Verification items for the finished model (mm, model axes). Face numbers are marked on the shaded views. A direction names the side the tool comes from. Give positions to 0.01 mm unless a question says otherwise; leave off trailing zeros. Write each loop counter-clockwise with the first axis right and the second up, starting at its lowest first coordinate (ties: lowest second). Pieces come first, ordered by that corner, then holes. Notation, with made-up numbers: (48.25, 7.25) - (91.25, 7.25) arc R13 ccw to (91.25, 16.25) - close; hole circle Ø7 at (-9, -1). An arc over 180 degrees is marked (long way). Put each result on its own line as item: value.
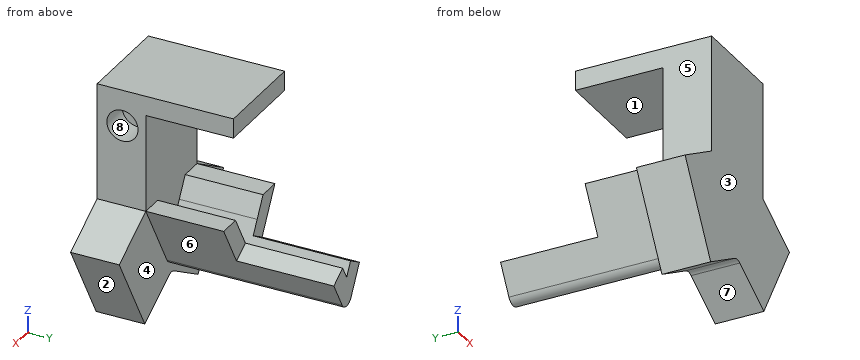
from build123d import *

# Parameters (mm, degrees)
BOSS_EXTRUDE1_DEPTH      = 2
BOSS_EXTRUDE1_DEPTH_BACK = 3
BOSS_EXTRUDE2_DEPTH      = 18
BOSS_EXTRUDE3_DEPTH      = 2
BOSS_EXTRUDE3_DEPTH_BACK = 3
SKETCH8_W                = 10
SKETCH8_H                = 12
SKETCH9_W                = 10
SKETCH9_H                = 2.002012711
BOSS_EXTRUDE4_DEPTH      = 18
CUT_EXTRUDE1_DEPTH       = 10
SKETCH12_W               = 10
SKETCH12_H               = 9
CUT_EXTRUDE3_DEPTH       = 3
FILLET3_R                = 1
FILLET4_R                = 1
SKETCH14_R               = 1.6
CUT_EXTRUDE4_DEPTH       = 3


with BuildPart() as part:
    # Sketch3 → Boss-Extrude1 (new, two sides: drawn at the far end of the back side and taken through both)
    with BuildSketch(Plane(origin=(0, 0, 0), x_dir=(1, 0, 0), z_dir=(0, 1, 0)).offset(-BOSS_EXTRUDE1_DEPTH_BACK)):
        Polygon((-16.281996431, 0), (-6.281996431, 0), (-1.085844009, 3), (-6.085844009, 11.660254038), (-11.281996431, 8.660254038), (-16.478148854, 11.660254038), (-21.478148854, 3), align=None)
    extrude(amount=BOSS_EXTRUDE1_DEPTH + BOSS_EXTRUDE1_DEPTH_BACK)

    # Sketch7 → Boss-Extrude2 (add)
    with BuildSketch(Plane(origin=(0, 2, 0), x_dir=(1, 0, 0), z_dir=(0, 1, 0))):
        Polygon((-6.281996431, 0), (-11.281996431, 8.660254038), (-16.281996431, 0), (-13.972595355, 0), (-12.817894816, 2), (-11.281996431, 4.660254038), (-9.746098047, 2), (-8.591397508, 0), align=None)
    extrude(amount=BOSS_EXTRUDE2_DEPTH)

    # Sketch8 → Boss-Extrude3 (add, two sides: drawn at the far end of the back side and taken through both)
    with BuildSketch(Plane(origin=(0, 0, 0), x_dir=(1, 0, 0), z_dir=(0, 1, 0)).offset(-BOSS_EXTRUDE3_DEPTH_BACK)):
        with Locations((-11.281996431, -6)):
            Rectangle(SKETCH8_W, SKETCH8_H)
    extrude(amount=BOSS_EXTRUDE3_DEPTH + BOSS_EXTRUDE3_DEPTH_BACK)

    # Sketch9 → Boss-Extrude4 (add)
    with BuildSketch(Plane(origin=(0, 2, 0), x_dir=(1, 0, 0), z_dir=(0, 1, 0))):
        with Locations((-11.281996431, -10.998993645)):
            Rectangle(SKETCH9_W, SKETCH9_H)
    extrude(amount=BOSS_EXTRUDE4_DEPTH)

    # Sketch10 → Cut-Extrude1 (cut)
    with BuildSketch(Plane(origin=(0, 20, 0), x_dir=(1, 0, 0), z_dir=(0, 1, 0))):
        Polygon((-13.781996431, 4.330127019), (-16.281996431, 0), (-13.972595355, 0), (-12.049945624, 3.330127019), align=None)
        Polygon((-6.281996431, 0), (-8.781996431, 4.330127019), (-10.514047239, 3.330127019), (-8.591397508, 0), align=None)
    extrude(amount=-CUT_EXTRUDE1_DEPTH, mode=Mode.SUBTRACT)

    # Sketch12 → Cut-Extrude3 (cut)
    with BuildSketch(Plane.XY.offset(12)):
        with Locations((-11.281996431, 15.5)):
            Rectangle(SKETCH12_W, SKETCH12_H)
    extrude(amount=-CUT_EXTRUDE3_DEPTH, mode=Mode.SUBTRACT)

    # Fillet3
    # the kernel refuses this fillet: 1 mm, written as the material it takes off along each edge
    with BuildSketch(Plane(origin=(-11.281996431, 2, -8.660254038), x_dir=(-0.5000000000000031, 0, 0.8660254037844368), z_dir=(0, 1, 0))) as fillet3_piece_1:
        with BuildLine():
            CenterArc((FILLET3_R * 1.73205080757, FILLET3_R), FILLET3_R, 150, 120)
            Line((FILLET3_R * 0.866025403784, FILLET3_R * 1.5), (0, 0))
            Line((0, 0), (FILLET3_R * 1.73205080757, 0))
        make_face()
    extrude(amount=22.330127019, mode=Mode.SUBTRACT)

    # Fillet4
    fillet4_edges = [part.edges().sort_by_distance(p)[0] for p in [
        (-11.281996431, -0.5, -8.660254038),
    ]]
    fillet(fillet4_edges, radius=FILLET4_R)

    # Sketch14 → Cut-Extrude4 (cut)
    with BuildSketch(Plane(origin=(-6.281996431, 0, 0), x_dir=(0, 0, -1), z_dir=(1, 0, 0))):
        with Locations((-8.29856454, -0.4)):
            Circle(SKETCH14_R)
    extrude(amount=-CUT_EXTRUDE4_DEPTH, mode=Mode.SUBTRACT)


solid = part.part
Q1. Scan lines: line 1 along Y through (x, z) = (-9.25, -8.5); line 2 along X through (y, z) = (12.25, -4.25); line 3 along Z through (x, y) = (-13.75, 4.25). Record each from-to range of solid material in increasing order.
Answers follow:
line 1: y = -3 to 2
line 2: x = -13.64 to -11.52, -11.05 to -8.92
line 3: z = -4.39 to -0.39, 10 to 12
Q2. Set-up check for the marked faces 4, 5, 6, 7 and 8: record each of +Z, -Z, +X, -X, +Y, -Y from which the full face is reachable in a straight line by a thin tool's end or side.
Answers follow:
face 4: -Z, +Y
face 5: +Z, -X, +Y, -Y
face 6: -Z, +X, +Y
face 7: -Z, +Y, -Y
face 8: +X
Q3. Section check B-B, the plane y = -0.4. Record the cut outline in (x, z).
Answers follow:
outline: (-21.48, -3) - (-16.48, -11.66) - (-11.78, -8.95) arc R1 cw to (-10.78, -8.95) - (-6.09, -11.66) - (-1.09, -3) - (-6.28, 0) - (-6.28, 6.7) - (-9.28, 6.7) - (-9.28, 9.9) - (-6.28, 9.9) - (-6.28, 12) - (-16.28, 12) - (-16.28, 0) - close
Q4. Section check C-C, the plane x = -15.75. Record the cut outline in (y, z), plus the area to 3 significant figures.
Answers follow:
outline: (-3, -11.24) - (2, -11.24) - (2, -0.92) - (10, -0.92) - (10, 0) - (2, 0) - (2, 10) - (11, 10) - (11, 12) - (-3, 12) - close
area: 142 mm2
Q5. Section check A-A, the plane y = 5.75. Record the cut outline in (x, z), plus the area to 3 significant figures.
Answers follow:
outline: (-16.28, 0) - (-12.15, -7.16) arc R1 ccw to (-10.42, -7.16) - (-6.28, 0) - (-8.59, 0) - (-11.28, -4.66) - (-13.97, 0) - close; (-16.28, 10) - (-6.28, 10) - (-6.28, 12) - (-16.28, 12) - close
area: 50.1 mm2
Q6. Go/stop test with flat-tipped pins: pin 1 Ø1.6 at (y, z) = (0.5, 9) entering from +X; pin 2 Ø10 at (x, y) = (-9, 7.5) entering from -Z; pin 3 Ø3.5 at (y, z) = (0.5, 5.5) entering from -X; pin 4 Ø4.5 at (x, z) = (-13.5, -2.5) entering from +Y. Record where each tip stops, or that it passes through.
Answers follow:
pin 1: stops at x = -6.28
pin 2: stops at z = -7.66
pin 3: stops at x = -16.28
pin 4: stops at y = 20
Q7. Release check for a two-part mould opening along Z. For the marked faces 1, 2 and 3 record: released by +Z, released by -Z, zero draft, split by the parting line, or undercut.
Answers follow:
face 1: undercut
face 2: released by -Z
face 3: zero draft
Q8. Section check D-D, the plane y = 10.5. Record the cut outline in (x, z).
Answers follow:
outline: (-16.28, 10) - (-6.28, 10) - (-6.28, 12) - (-16.28, 12) - close; (-13.78, -4.33) - (-12.15, -7.16) arc R1 ccw to (-10.42, -7.16) - (-8.78, -4.33) - (-10.51, -3.33) - (-11.28, -4.66) - (-12.05, -3.33) - close
